Autodesk Inventor part; units mm, degrees
ref_plane "YZ Plane" through (0, 0, 0) normal (1, 0, 0) x (0, 1, 0)
ref_plane "XZ Plane" through (0, 0, 0) normal (0, 1, 0) x (-1, 0, 0)
ref_plane "XY Plane" through (0, 0, 0) normal (0, 0, 1) x (1, 0, 0)
sketch "Sketch1" plane through (0, 0, 0) normal (0, 0, 1) x (1, 0, 0)
  line L0 (0, 0) -> (12.7, 0)
  line L1 (12.7, 0) -> (12.7, 23.622)
  line L2 (12.7, 23.622) -> (0, 23.622)
  line L3 (0, 23.622) -> (0, 0)
  dimension "d0" = 12.7
  dimension "d1" = 23.622
extrude "Extrusion1" add sketch "Sketch1" along normal blind 6.35
sketch "Sketch2" plane through (0, 0, 6.35) normal (0, 0, 1) x (1, 0, 0)
  line L0 (12.7, 0) -> (12.7, 23.622)
  line L1 (0, 0) -> (12.7, 0)
  point P0 (6.35, 7.62)
  dimension "d4" = 6.35
  dimension "d5" = 7.62
hole "6 MM Hole" at (6.35, 7.62, 6.35) direction (0, 0, -1) diameter 4.9276 end through all countersink diameter 6.35 countersink angle 90
sketch "Sketch3" plane through (0, 23.622, 0) normal (0, 1, 0) x (1, 0, 0)
  line L0 (12.7, 0) -> (0, 0)
  line L1 (0, 0) -> (0, -6.35)
  point P0 (6.35, -3.175)
  dimension "d13" = 3.175
  dimension "d14" = 6.35
hole "Hole2" at (6.35, 23.622, 3.175) direction (0, -1, 0) diameter 3.2512 depth 12.065 tip angle 118 countersink diameter 4.064 countersink angle 90
chamfer "Chamfer1" distance 0.508 angle 45 1 edges at (6.35, 10.0838, 0)
properties part number "Rear Leg"
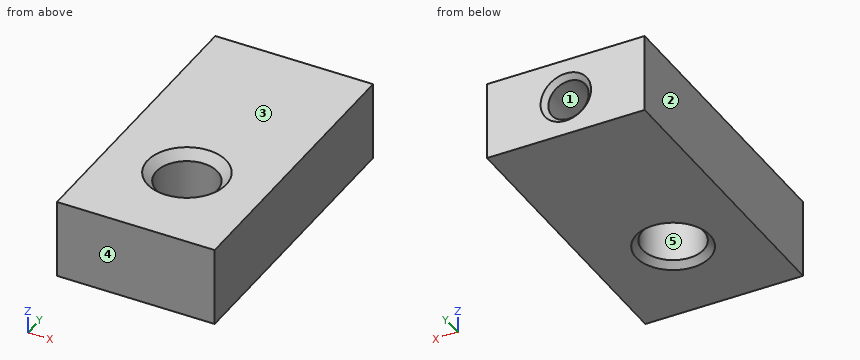
Geometry check sheet. Reference: the model listing, model coordinates, mm. Face numbers are marked on the shaded views. A direction names the side the tool comes from. Coordinates: 2 decimals unless noted, no trailing zeros. Order: outer loops, then holes, each group sorted by start corner. A loop starts at its lowest first (then second) coordinate and runs counter-clockwise, first axis right, second up. Notation, with made-up numbers: (75, -32.75) - (108, -32.75) arc R13 ccw to (108, -24.75) - close; hole circle Ø7 at (65.5, 64.5). An arc over 180 degrees is marked (long way). Answer as a JSON object with one key per item and string values. Group by question number.
Item 1: Tool access check on the marked faces 1 and 2. Record the directions out of +Z, -Z, +X, -X, +Y, -Y that give a thin tool (end or side, any length) a straight path to the whole face; none if there is none.
Item 2: Sectioned sample at C-C, the plane z = 6. Record the cut outline in (x, y) (3 decimals), and give its area (3 significant figures).
Item 3: Draft check along Y on the marked faces 3, 4 and 5. Enter one of: +Y half, -Y half, draft (parallel to the pull), parting line (faces both ways), or undercut.
Item 4: Sectioned sample at B-B, the plane y = 17.25. Record the cut outline in (x, z) (3 decimals).
Item 5: Sectioned sample at A-A, the plane y = 7.62. Record the cut outline in (x, z) (3 decimals).
Item 6: Scan lines: probe 1 along X at (y, z) = (19, 3.25); probe 2 along Y at (x, z) = (8.25, 2.5); probe 3 along X at (y, z) = (14.75, 4.5). Record each from-to range of solid material in increasing order.
Resolved:
{
 "1": {"face 1": "+Y", "face 2": "+Z, -Z, -X, +Y, -Y"},
 "2": {"outline": "(0, 0) - (12.7, 0) - (12.7, 23.622) - (0, 23.622) - close; hole circle Ø5.65 at (6.35, 7.62)", "area": "275 mm^2"},
 "3": {"face 3": "draft", "face 4": "-Y half", "face 5": "undercut"},
 "4": {"outline": "(0, 0) - (12.7, 0) - (12.7, 6.35) - (0, 6.35) - close; hole circle Ø3.251 at (6.35, 3.175)"},
 "5": {"outline": "(0, 0) - (3.378, 0) - (3.886, 0.508) - (3.886, 5.639) - (3.175, 6.35) - (0, 6.35) - close; (8.814, 0.508) - (9.322, 0) - (12.7, 0) - (12.7, 6.35) - (9.525, 6.35) - (8.814, 5.639) - close"},
 "6": {"probe 1": "0 to 4.73, 7.97 to 12.7", "probe 2": "0 to 6.05, 9.19 to 23.61", "probe 3": "0 to 5.41, 7.29 to 12.7"}
}
